Build history of the part. All positions in model axes, mm. A direction names the side the tool comes from. Round coordinates to 2 decimals unless told otherwise and drop trailing zeros. Write each loop counter-clockwise with the first axis right and the second up, starting at its lowest first coordinate (ties: lowest second). Pieces come first, ordered by that corner, then holes. Notation, with made-up numbers: (81.5, -38.5) - (96.5, -38.5) arc R28 cw to (96.5, -12.5) - close; hole circle Ø8 at (15, -12). An arc over 180 degrees is marked (long way). Answer as a JSON object with one key per item and string values. Group by question number.
Item 1: Slice it at C-C, the plane z = 25. List the corners of the cut face in (x, y) (3 decimals), then the cut area to 3 significant figures.
Item 2: Which spindle directions (+Z, -Z, +X, -X, +Y, -Y) get a long thin tool onto all of the face, cutting with end or side? Do faces 1 (the flat face through (-33, 15, 1)), 2 (the flat face through (-31, 17.5, -1)), 3 (the flat face through (2.8, 6.2, 15)), 4 (the cylindrical face through (-19.97, 23.16, -1.01)). Say none if no direction does.
Item 3: Slice it at D-D, the plane y = 0. Give the number of separate pieces and of enclosed holes in the cut face, then the cut area to 4 significant figures.
Item 4: Two-plate mould, pull along Y, no slides. Class faces 5 (the flat face through (-26, 27.5, -1)), 6 (the flat face through (-37.5, 23, -1)), 7 (the flat face through (-27, 26.5, -1)): +Y half, -Y half, draft (parallel to the pull), parting line (faces both ways), or undercut.
Item 5: Slice it at A-A, the plane x = -31.5. List the corners of the cut face in (y, z), then the cut area to 3 significant figures.
Item 6: Probe line 1 (Y direction, x = 0, z = 21.5) (3 decimals); line 2 (Y direction, x = 0, z = 0.4); line 3 (Z direction, x = -11, y = 0.5). List the from-to ranges inside material, lowest first. Write a range as from..to.
Item 7: Flat gauge pins, fed straight in: pin 1 (4 mm diameter, centred on x = -7, z = 5, fed in from +Y); pin 2 (1 mm diameter, centred on x = 0, y = -23, fed in from -Z); pin 3 (22.5 mm diameter, centred on x = 0, y = 0, fed in from +Z); pin 4 (8 mm diameter, centred on y = 13.5, z = 28.5, fed in from -X). Where does each tip first touch, or does it go through?
Item 8: Slice it at B-B, the plane y = -31.5. List the corners of the cut face in (x, z).
Autodesk Fusion 360 part; units mm, degrees
sketch "Skizze1" plane through (0, 0, 0) normal (0, 0, 1) x (1, 0, 0)
  line L0 (-40, 17) -> (0, 17)
  line L1 (0, 30) -> (-40, 30)
  line L2 (-40, 15) -> (0, 15)
  circle A0 centre (0, 31.5) radius 2
  line L3 (-40, 28) -> (0, 28)
  circle A1 centre (0, 0) radius 30
  circle A2 centre (0, 31.5) radius 1
  line L4 (0, 15) -> (0, 30)
  line L5 (-40, 15) -> (-40, 17)
  line L6 (-40, 30) -> (-40, 15)
  circle A3 centre (-31.5, 0) radius 1
  circle A4 centre (0, -31.5) radius 2
  circle A5 centre (31.5, 0) radius 2
  circle A6 centre (31.5, 0) radius 1
  circle A7 centre (0, 0) radius 28
  circle A8 centre (0, -31.5) radius 1
  line L7 (-40, 30) -> (-40, 28)
  circle A9 centre (-31.5, 0) radius 2
  line L8 (-38, 28) -> (-38, 17)
  line L9 (-38, 27.5) -> (-37.5, 27.5)
  line L10 (-37.5, 27.5) -> (-37.5, 17.5)
  line L11 (-37.5, 17.5) -> (-25, 17.5)
  line L12 (-37.5, 27.5) -> (-13.5, 27.5)
  arc A10 (-13.5, 27.5) -> (-25, 17.5) centre (0.0202, 0.3392) ccw
  line L13 (-36.5, 26.5) -> (-17.5, 26.5)
  line L14 (-36.5, 26.5) -> (-36.5, 18.5)
  line L15 (-36.5, 18.5) -> (-26, 18.5)
  arc A11 (-17.5, 26.5) -> (-26, 18.5) centre (-0.9044, 0.3515) ccw
  circle A12 centre (0, 0) radius 27.75
  circle A13 centre (0, 0) radius 26.75
  circle A14 centre (0, 0) radius 6.625
  circle A15 centre (0, 0) radius 5.375
  circle A16 centre (0, 0) radius 12.5
  circle A17 centre (0, 0) radius 13.5
  dimension "d1" = 60
  dimension "d7" = 2
  dimension "d8" = 4
  dimension "d9" = 2
  dimension "d10" = 4
  dimension "d11" = 2
  dimension "d12" = 4
  dimension "d13" = 2
  dimension "d14" = 4
  dimension "d15" = 40
  dimension "d16" = 15
  dimension "d17" = 2
  dimension "d18" = 56
  dimension "d19" = 2
  dimension "d20" = 0.5
  dimension "d21" = 55.5
  dimension "d22" = 53.5
  dimension "d29" = 13.25
  dimension "d30" = 10.75
  dimension "d39" = 25
  dimension "d40" = 27
extrude "Extrusion3" add sketch "Skizze1" along normal blind 2 contours L0 L3 L6 L8 | L0 L2 A1 L5 L6 | L0 L3 A1 L8 | L1 A0 L3 A1 L6 L7 | L0 L3 A1 A7 | L0 L2 A1 A7 | L2 A0 A1 L4 A4 A5 A7 A9 | L0 L4 A7 A12 | L0 L2 A7 A12 | A0 L3 A1 L4 | L2 L4 A7 A12 | A1 A9 | A1 A9 | L1 A0 A1 | L1 A0 A1 | A0 A1 L4 | A0 A1 L4 | L0 L4 A13 | L0 L2 L4 A13 | L2 L4 A13 | A1 A4 | A1 A4 | A1 A5 | A1 A5 | L13 L14 L15 A11 makes body 1 at (-33, 21.1667, 0) makes body 2 at (-34.4936, 15.8333, 2) makes body 3 at (22.1835, -1.9997, 0)
extrude "Extrusion4" add sketch "Skizze1" along normal blind 2 and the other way blind 2 contours L10 L11 L12 A10 | L0 L4 A12 A13 | L0 L2 A12 A13 | L2 L4 A12 A13 bodies 1 2 3
extrude "Extrusion6" add sketch "Skizze1" along normal blind 15 contours A17 bodies 1
extrude "Extrusion7" add sketch "Skizze1" along normal blind 2 from surface at 13 contours A16 bodies 1
extrude "Extrusion8" add sketch "Skizze1" along normal blind 20 from surface at 13 contours A14 bodies 1
Geometry says:
{
 "1": {"outline": "circle Ø13.25 at (0, 0); hole circle Ø10.75 at (0, 0)", "area": "47.1 mm^2"},
 "2": {"face 1": "+Z, -Z, -X", "face 2": "-Z, -X", "face 3": "+Z", "face 4": "-Z"},
 "3": {"separate pieces": "4", "enclosed holes": "0", "area": "179.5 mm^2"},
 "4": {"face 5": "+Y half", "face 6": "draft", "face 7": "undercut"},
 "5": {"outline": "(-2, 0) - (-1, 0) - (-1, 2) - (-2, 2) - close; (1, 0) - (2, 0) - (2, 2) - (1, 2) - close; (15, 0) - (17.5, 0) - (17.5, -2) - (18.5, -2) - (18.5, 0) - (26.5, 0) - (26.5, -2) - (27.5, -2) - (27.5, 0) - (30, 0) - (30, 2) - (15, 2) - close", "area": "38.0 mm^2"},
 "6": {"line 1": "y = -6.625..-5.375, 5.375..6.625", "line 2": "y = -33.5..-32.5, -30.5..-12.5, 12.5..30.5, 32.5..33.5", "line 3": "z = 13..15"},
 "7": {"pin 1": "stops at y = 12.54", "pin 2": "stops at z = 0", "pin 3": "stops at z = 33", "pin 4": "passes through"},
 "8": {"outline": "(-2, 0) - (-1, 0) - (-1, 2) - (-2, 2) - close; (1, 0) - (2, 0) - (2, 2) - (1, 2) - close"}
}
